Check sheet for the modelled part. Datum: model origin and axes. Units: mm. Face numbers are marked on the shaded views. A direction names the side the tool comes from. Round coordinates to 2 decimals unless told otherwise and drop trailing zeros. Loops run counter-clockwise (first coordinate to the right, second up) from the corner with the lowest first, then second, coordinate; pieces in that order, holes last. Notation, with made-up numbers: (-28.5, -25.75) -> (-15.5, -25.75) arc R18 cw to (-15.5, -15.75) -> close; hole circle Ø7 at (15, 72). An arc over 180 degrees is marked (long way). One line per item, written item: value. Start each with the question number.
1. Cross-section at C-C on z = 0. Record the cut outline in (x, y), then the cut area to 3 significant figures.
2. Material ranges on L1, parallel to Y at x = 3, z = -11; L2, parallel to Z at x = 1.5, y = 4.75; L3, parallel to Z at x = -4.5, y = 7.5, recorded low to high.
3. Cross-section at B-B on x = 0. Record the cut outline in (y, z), then the cut area to 3 significant figures.
4. Go/stop test with flat-tipped pins: pin 1 (3 mm diameter, centred on x = -9, z = -9, fed in from +Y); pin 2 (1 mm diameter, centred on y = 8, z = 5, fed in from +X); pin 3 (1 mm diameter, centred on y = 7, z = 5.5, fed in from -X); pin 4 (5 mm diameter, centred on y = 5, z = 8.5, fed in from -X). Record where each tip stops, or that it passes through.
5. Cross-section at A-A on y = 7. Record the cut outline in (x, z) (3 decimals).
6. Cross-section at D-D on y = 1.25. Record the cut outline in (x, z), then the cut area to 3 significant figures.
7. Set-up check for the marked faces 1 and 2: record each of +Z, -Z, +X, -X, +Y, -Y from which the full face is reachable in a straight line by a thin tool's end or side.
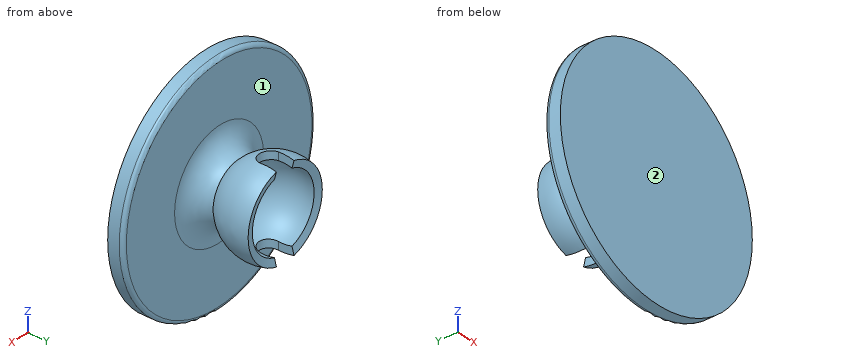
from build123d import *

# Parameters (mm, degrees)
SKETCH3_R               = 15
BOSS_EXTRUDE1_DEPTH     = 2
CUT_EXTRUDE1_DEPTH      = 23.872523746
CUT_EXTRUDE1_DEPTH_BACK = 23.872523746
FILLET1_R               = 3
FILLET2_R               = 0.5


with BuildPart() as part:
    # Sketch2 → Revolve2 (revolve)
    with BuildSketch(Plane.XY):
        with BuildLine():
            Line((0, 0), (4, 0))
            Line((4, 0), (4, 2.527864045))
            ThreePointArc((4, 2.527864045), (5.75008972, 5.28638738), (5.795554958, 8.552914271))
            Line((5.795554958, 8.552914271), (4.829629131, 8.294095226))
            ThreePointArc((4.829629131, 8.294095226), (3.966766701, 3.956192855), (0, 2))
            Line((0, 2), (0, 0))
        make_face()
    revolve(axis=Axis((0, 2, 0), (0, -1, 0)))

    # Sketch3 → Boss-Extrude1 (add)
    with BuildSketch(Plane.XZ):
        Circle(SKETCH3_R)
    extrude(amount=BOSS_EXTRUDE1_DEPTH)

    # Sketch6 → Cut-Extrude1 (cut, two sides: drawn at the far end of the back side and taken through both)
    with BuildSketch(Plane.XY.offset(-CUT_EXTRUDE1_DEPTH_BACK)):
        with BuildLine():
            Line((1.375, 6.552914271), (1.375, 8.552914271))
            Line((1.375, 8.552914271), (-1.375, 8.552914271))
            Line((-1.375, 8.552914271), (-1.375, 6.552914271))
            ThreePointArc((-1.375, 6.552914271), (0, 5.177914271), (1.375, 6.552914271))
        make_face()
    extrude(amount=CUT_EXTRUDE1_DEPTH + CUT_EXTRUDE1_DEPTH_BACK, mode=Mode.SUBTRACT)

    # Fillet1
    # the kernel refuses this fillet: 3 mm, written as the material it adds along each edge
    with BuildSketch(Plane(origin=(0, 0, 0), x_dir=(1, 0, 0), z_dir=(0, 0, -1))) as fillet1_piece_1:
        with BuildLine():
            CenterArc((6.962615, -3), FILLET1_R, 90, 80.945223599)
            Line((4, -2.527864045), (3.9407477, -2.518421326))
            ThreePointArc((3.9407477, -2.518421326), (3.94, -1.263932023), (3.94, 0))
            Line((3.94, 0), (4, 0.06))
            Line((4, 0.06), (6.962615, 0.06))
            Line((6.962615, 0.06), (6.962615, 0))
        make_face()
    revolve(axis=Axis((0, 0, 0), (0, -1, 0)))

    # Fillet2
    fillet2_edges = [part.edges().sort_by_distance(p)[0] for p in [
        (-15, 0, 0),
    ]]
    fillet(fillet2_edges, radius=FILLET2_R)


solid = part.part
Taken from the geometry:
1. outline: (-15, -2) -> (15, -2) -> (15, -0.5) arc R0.5 ccw to (14.5, 0) -> (6.96, 0) arc R3 cw to (4, 2.53) arc R6 ccw to (5.8, 8.55) -> (4.83, 8.29) arc R5 cw (long way) to (-4.83, 8.29) -> (-5.8, 8.55) arc R6 ccw to (-4, 2.53) arc R3 cw to (-6.96, 0) -> (-14.5, 0) arc R0.5 ccw to (-15, -0.5) -> close
1. area: 95.6 mm2
2. L1: y = -2 to 0
2. L2: z = -5.36 to -4.21, 4.21 to 5.36
2. L3: z = -3.94 to -2.12, 2.12 to 3.94
3. outline: (-2, -15) -> (-0.5, -15) arc R0.5 ccw to (0, -14.5) -> (0, -6.96) arc R3 cw to (2.53, -4) arc R6 ccw to (5.18, -5.72) -> (5.18, -4.66) arc R5 cw to (5.18, 4.66) -> (5.18, 5.72) arc R6 ccw to (2.53, 4) arc R3 cw to (0, 6.96) -> (0, 14.5) arc R0.5 ccw to (-0.5, 15) -> (-2, 15) -> close
3. area: 89.0 mm2
4. pin 1: stops at y = 0
4. pin 2: stops at x = 3.85
4. pin 3: stops at x = -3.32
4. pin 4: passes through
5. outline: (-1.375, -5.84) -> (-1.375, -4.807) arc R5 cw to (-1.375, 4.807) -> (-1.375, 5.84) arc R6 ccw to start; (1.375, -5.84) arc R6 ccw to (1.375, 5.84) -> (1.375, 4.807) arc R5 cw to (1.375, -4.807) -> close
6. outline: circle Ø9.05 at (0, 0)
6. area: 64.4 mm2
7. face 1: +Y
7. face 2: +Z, -Z, +X, -X, -Y
